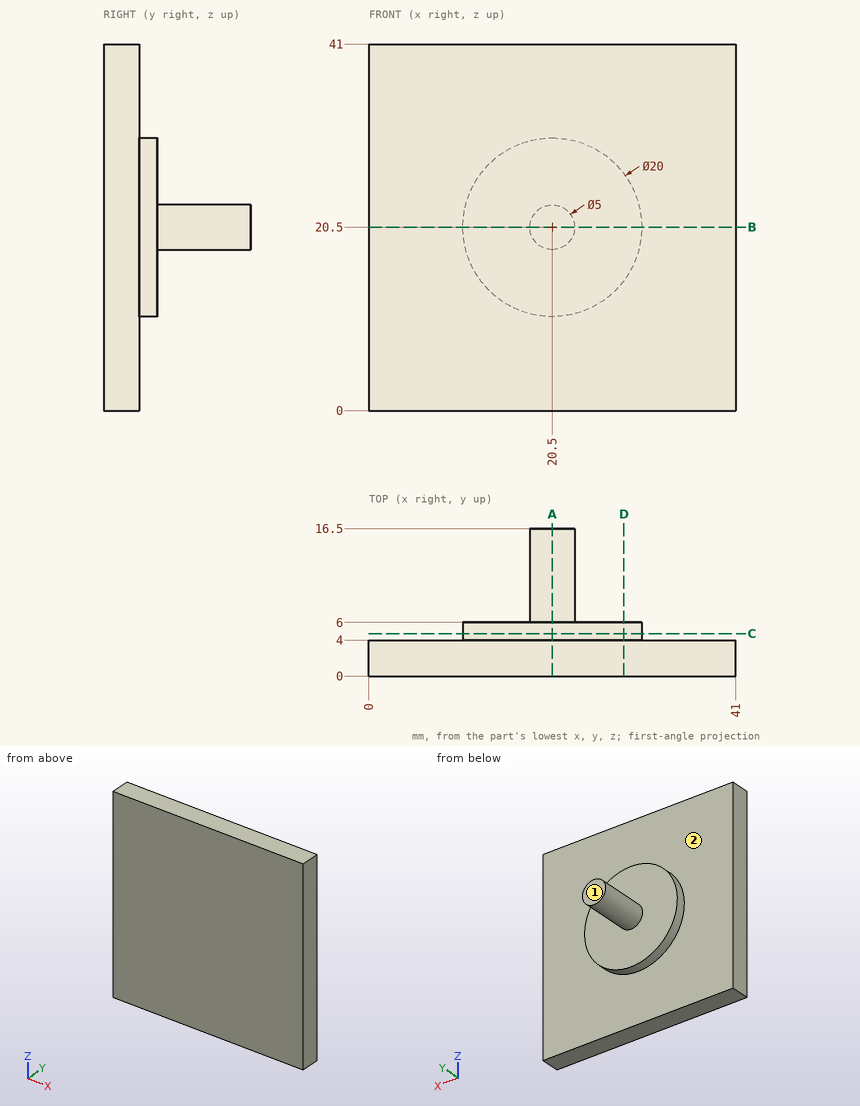
Source: three-view drawing plus pictorial views. Frame: mm from the lowest corner of the part. A direction names the side the tool comes from. Give positions to 0.01 mm unless a question says otherwise; leave off trailing zeros. Loops run counter-clockwise (first coordinate to the right, second up) from the corner with the lowest first, then second, coordinate; pieces in that order, holes last. Notation, with made-up numbers: (54.25, 32.5) -> (67.25, 32.5) arc R5 cw to (67.25, 41.5) -> close; hole circle Ø5 at (37, 23). An arc over 180 degrees is marked (long way). Put each result on its own line as item: value. Start each with the question number.
1) Reachability of the marked faces 1 and 2 from +Z, -Z, +X, -X, +Y, -Y: full face, straight path, thin tool, end or side. Return the list, or none.
2) Contact query for flat-ended pins moving along their axis: P1, Ø5, axis at x = 19, y = 10, coming from the +Z side; P2, Ø3, axis at x = 22.5, z = 6.5, coming from the +Y side; P3, Ø1.5, axis at x = 27, y = 8.5, coming from the +Z side. Output: stop coordinate, or through.
3) Cut plane D-D (x = 28.5). Return loops of the section in (y, z).
4) Cut plane B-B (z = 20.5). Return loops of the section in (x, y).
5) Cut plane C-C (y = 4.75). Return loops of the section in (x, z), then the cut area to 3 significant figures.
6) Cut plane A-A (x = 20.5). Return loops of the section in (y, z), then the cut area to 4 significant figures.
7) Material intervals for probe 1 along Y at (x, z) = (31, 10.5); probe 2 along Z at (x, y) = (20, 9.25), sorted ascending.
Results are:
1. face 1: +Z, -Z, +X, -X, +Y
1. face 2: +Y
2. P1: stops at z = 23
2. P2: stops at y = 4
2. P3: passes through
3. outline: (0, 0) -> (4, 0) -> (4, 14.5) -> (6, 14.5) -> (6, 26.5) -> (4, 26.5) -> (4, 41) -> (0, 41) -> close
4. outline: (0, 0) -> (41, 0) -> (41, 4) -> (30.5, 4) -> (30.5, 6) -> (23, 6) -> (23, 16.5) -> (18, 16.5) -> (18, 6) -> (10.5, 6) -> (10.5, 4) -> (0, 4) -> close
5. outline: circle Ø20 at (20.5, 20.5)
5. area: 314 mm2
6. outline: (0, 0) -> (4, 0) -> (4, 10.5) -> (6, 10.5) -> (6, 18) -> (16.5, 18) -> (16.5, 23) -> (6, 23) -> (6, 30.5) -> (4, 30.5) -> (4, 41) -> (0, 41) -> close
6. area: 256.5 mm2
7. probe 1: y = 0 to 4
7. probe 2: z = 18.05 to 22.95
